Here's how the part is built. I have some questions about the finished solid (model axes, mm). A direction names the side the tool comes from. Give positions to 0.01 mm unless a question says otherwise; leave off trailing zeros. Write each loop counter-clockwise with the first axis right and the second up, starting at its lowest first coordinate (ties: lowest second). Pieces come first, ordered by that corner, then holes. Notation, with made-up numbers: (52.25, 23) - (101.25, 23) arc R13 cw to (101.25, 35) - close; hole circle Ø10 at (27.25, 12). An arc over 180 degrees is marked (long way). Use a Markdown table: item, result.
```python
from build123d import *

# Parameters (mm, degrees)
SKETCH1_R           = 41
BOSS_EXTRUDE1_DEPTH = 265
SKETCH2_OUTSIDE_W   = 141.852
SKETCH2_OUTSIDE_H   = 141.852
SKETCH2_OUTSIDE_R   = 13
CUT_EXTRUDE1_DEPTH  = 25
CHAMFER1_SIZE2      = 28
CHAMFER1_SIZE       = 51
CUT_EXTRUDE2_START  = -32
SKETCH3_OUTSIDE_W   = 141.852
SKETCH3_OUTSIDE_H   = 141.852
SKETCH3_OUTSIDE_R   = 38
CUT_EXTRUDE2_DEPTH  = 64
CHAMFER2_SIZE2      = 38
CHAMFER2_SIZE       = 3
CHAMFER3_SIZE2      = 3
CHAMFER3_SIZE       = 12
CHAMFER4_SIZE2      = 8
CHAMFER4_SIZE       = 32
FILLET1_R           = 5
FILLET2_R           = 15


with BuildPart() as part:
    # Sketch1 → Boss-Extrude1 (new body)
    with BuildSketch(Plane(origin=(0, 0, 0), x_dir=(1, 0, 0), z_dir=(0, 1, 0))):
        with Locations(Location((0, 0, 0), (0, 0, 270))):
            Circle(SKETCH1_R)
    extrude(amount=BOSS_EXTRUDE1_DEPTH)

    # Sketch2 outside → Cut-Extrude1 (cut)
    with BuildSketch(Plane(origin=(0, 265, 0), x_dir=(1, 0, 0), z_dir=(0, 1, 0))):
        Rectangle(SKETCH2_OUTSIDE_W, SKETCH2_OUTSIDE_H)
        with Locations(Location((0, 0, 0), (0, 0, 270))):
            Circle(SKETCH2_OUTSIDE_R, mode=Mode.SUBTRACT)
    extrude(amount=-CUT_EXTRUDE1_DEPTH, mode=Mode.SUBTRACT)

    # Chamfer1
    chamfer1_edges = [part.edges().sort_by_distance(p)[0] for p in [
        (0, 240, -41),
    ]]
    chamfer1_side = [part.faces().sort_by_distance(p)[0] for p in [
        (0, 239.44, -41),
    ]]
    chamfer(chamfer1_edges, length=CHAMFER1_SIZE - 0.0001, length2=CHAMFER1_SIZE2 - 0.0001, reference=chamfer1_side[0])  # a hair under: the kernel refuses the full size

    # Sketch3 outside → Cut-Extrude2 (cut)
    with BuildSketch(Plane.XZ.offset(CUT_EXTRUDE2_START)):
        Rectangle(SKETCH3_OUTSIDE_W, SKETCH3_OUTSIDE_H)
        with Locations(Location((0, 0, 0), (0, 0, 270))):
            Circle(SKETCH3_OUTSIDE_R, mode=Mode.SUBTRACT)
    extrude(amount=-CUT_EXTRUDE2_DEPTH, mode=Mode.SUBTRACT)

    # Chamfer2
    chamfer2_edges = [part.edges().sort_by_distance(p)[0] for p in [
        (0, 32, 38),
    ]]
    chamfer2_side = [part.faces().sort_by_distance(p)[0] for p in [
        (0, 32, 38.06),
    ]]
    chamfer(chamfer2_edges, length=CHAMFER2_SIZE - 0.0001, length2=CHAMFER2_SIZE2 - 0.0001, reference=chamfer2_side[0])  # a hair under: the kernel refuses the full size

    # Chamfer3
    chamfer3_edges = [part.edges().sort_by_distance(p)[0] for p in [
        (0, 96, 38),
    ]]
    chamfer3_side = [part.faces().sort_by_distance(p)[0] for p in [
        (0, 95.94, 38),
    ]]
    chamfer(chamfer3_edges, length=CHAMFER3_SIZE - 0.0001, length2=CHAMFER3_SIZE2 - 0.0001, reference=chamfer3_side[0])  # a hair under: the kernel refuses the full size

    # Chamfer4
    chamfer4_edges = [part.edges().sort_by_distance(p)[0] for p in [
        (0, 0, -41),
    ]]
    chamfer4_side = [part.faces().sort_by_distance(p)[0] for p in [
        (0, 0.16, -41),
    ]]
    chamfer(chamfer4_edges, length=CHAMFER4_SIZE - 0.0001, length2=CHAMFER4_SIZE2 - 0.0001, reference=chamfer4_side[0])  # a hair under: the kernel refuses the full size

    # Fillet1
    fillet1_edges = [part.edges().sort_by_distance(p)[0] for p in [
        (0, 0, -33.0001),
    ]]
    fillet(fillet1_edges, radius=FILLET1_R)

    # Fillet2
    fillet2_edges = [part.edges().sort_by_distance(p)[0] for p in [
        (0, 189.0001, -41),
    ]]
    fillet(fillet2_edges, radius=FILLET2_R)


solid = part.part
```
Item 1: Thinking about a two-plate mould opening in Y: for faces 1 (the flat face through (0, 0, 0)), 2 (the conical face through (11.471, 84.751, -36.424)), 3 (the conical face through (19.603, 227.103, -4.353)), which applies, +Y half, -Y half, draft (parallel to the pull), parting line (faces both ways), or undercut?
Values:
| item | result |
|---|---|
| face 1 | -Y half |
| face 2 | undercut |
| face 3 | +Y half |
Item 2: If we section it at A-A, the plane y = 109.5: Write out the boundary of the cut face in (x, z), plus the area to 3 significant figures.
Values:
| item | result |
|---|---|
| outline | circle Ø82 at (0, 0) |
| area | 5,280 mm2 |
Item 3: For faces 4 (the cylindrical face through (-40, 140, -9)), 5 (the cylindrical face through (-7.91, 252.675, -10.316)), 6 (the conical face through (-23.82, 55.488, 31.065)), which set-ups out of +Z, -Z, +X, -X, +Y, -Y let a thin tool reach every point of the face, with its end or its side?
Values:
| item | result |
|---|---|
| face 4 | +Y, -Y |
| face 5 | +Y |
| face 6 | none |
Item 4: I need wall thicknesses on line 1 along Z through (x, y) = (1, 163.5); line 2 along Z through (x, y) = (17, 70.5). Which ranges of each line are inside material? Lowest first, please. Write a range as [from, to].
Values:
| item | result |
|---|---|
| line 1 | z = [-40.99, 40.99] |
| line 2 | z = [-33.99, 33.99] |
Item 5: Will these pins go through, and if not, where does the flat tip stop? pin 1 Ø1.5 at (y, z) = (106.5, -14) entering from -X; pin 2 Ø1.5 at (x, z) = (-15, 2) entering from +Y; pin 3 Ø3 at (y, z) = (142.5, -19.5) entering from -X.
Values:
| item | result |
|---|---|
| pin 1 | stops at x = -38.8 |
| pin 2 | stops at y = 237.48 |
| pin 3 | stops at x = -36.84 |
